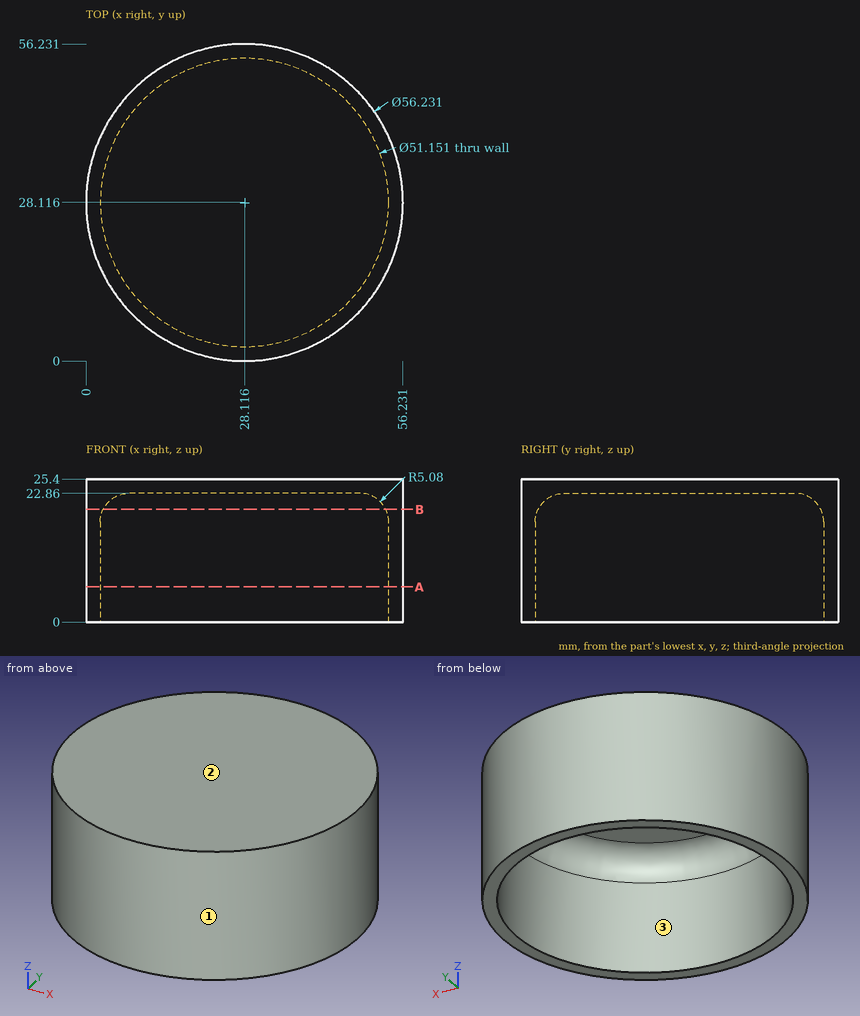
Part print with two shaded views. Sizes in mm from the minimum x, y, z corner. Give positions to 0.01 mm unless a question says otherwise; leave off trailing zeros. Loops run counter-clockwise (first coordinate to the right, second up) from the corner with the lowest first, then second, coordinate; pieces in that order, holes last. Notation, with made-up numbers: (-7.5, 16) - (-2.5, 16) arc R28 cw to (-2.5, 46) - close; hole circle Ø11 at (-24, 2.25). An arc over 180 degrees is marked (long way). Put each result on its own line as item: value.
Q1. Mould opens along X. For the marked faces 1, 2 and 3 say: pulls with the +X half, pulls with the -X half, needs draft (parallel to the pull), parting line crosses it, or undercut.
Filled in:
face 1: parting line crosses it
face 2: needs draft
face 3: undercut
Q2. Flat gauge pins, fed straight in: pin 1 (3 mm diameter, centred on y = 39.5, z = 6, fed in from +X); pin 2 (1.5 mm diameter, centred on y = 21.5, z = 19, fed in from -X); pin 3 (6 mm diameter, centred on x = 26, z = 16, fed in from -Y). Where does each tip first touch, or does it go through?
Filled in:
pin 1: stops at x = 54.44
pin 2: stops at x = 0.62
pin 3: stops at y = 0
Q3. Probe line 1 along X through (y, z) = (28.5, 7); line 2 along Z through (x, y) = (18, 16); line 3 along Y through (x, z) = (13, 6.75) (1 decimal). List the from-to ranges inside material, lowest first.
Filled in:
line 1: x = 0 to 2.54, 53.69 to 56.23
line 2: z = 22.86 to 25.4
line 3: y = 4.4 to 7.5, 48.7 to 51.8
Q4. Slice it at B-B (z = 20). Give the cut face in (x, y) (1 decimal).
Filled in:
outline: circle Ø56.2 at (28.1, 28.1); hole circle Ø50.1 at (28.1, 28.1)
Q5. Slice it at A-A (z = 6.25). Give the cut face in (x, y) (1 decimal).
Filled in:
outline: circle Ø56.2 at (28.1, 28.1); hole circle Ø51.2 at (28.1, 28.1)
